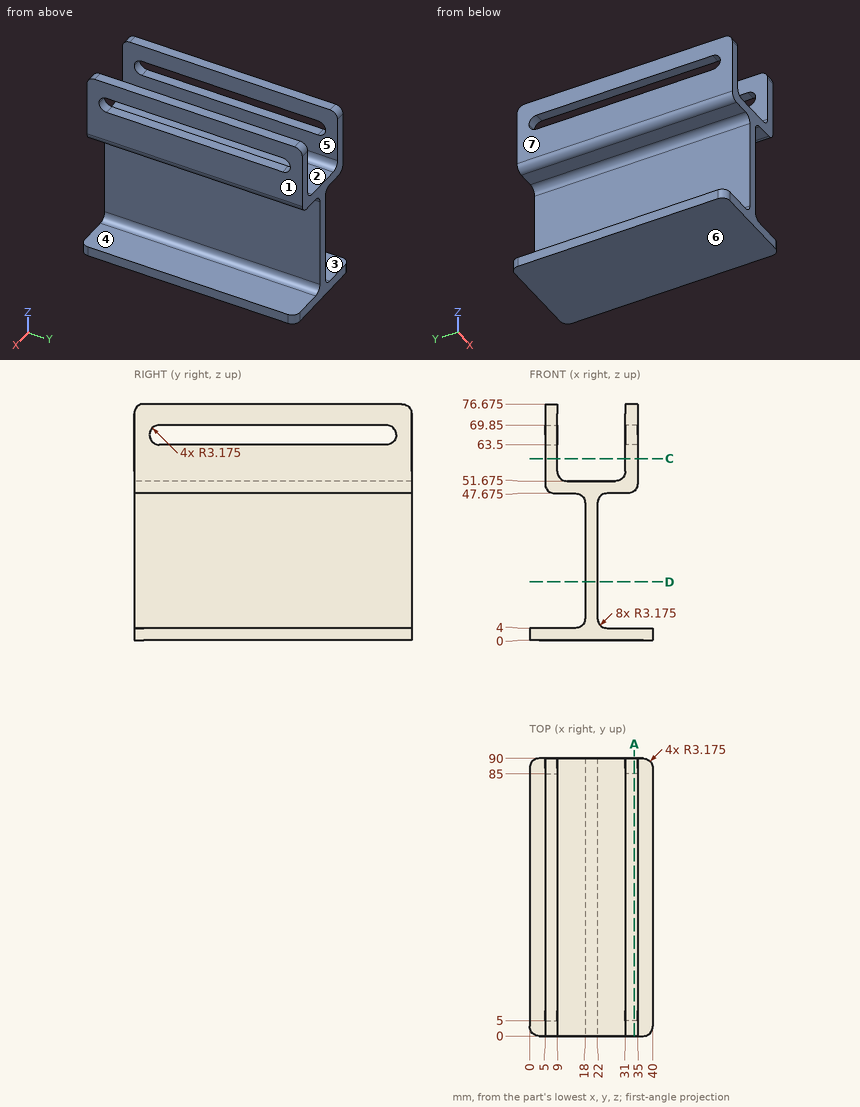
Here's the drawing with two shaded views (mm, measured from the low corner). I have some questions. A direction names the side the tool comes from. Give positions to 0.01 mm unless a question says otherwise; leave off trailing zeros. Loops run counter-clockwise (first coordinate to the right, second up) from the corner with the lowest first, then second, coordinate; pieces in that order, holes last. Notation, with made-up numbers: M 63,84 L 120,84 A12 ccw 120,96 Z; hole C 78.25,-13.5 d3. An arc over 180 degrees is marked long. One line per item, written item: value. Start each with the question number.
1) If we section it at D-D, the plane z = 19: Write out the boundary of the cut face in (x, y).
2) If I drill on line 1 (X direction, y = 19, z = 57); line 2 (Z direction, x = 27, y = 66) (3 decimals); line 3 (Z direction, x = 5.5, y = 29) (3 decimals), over which ranges is the centre line in solid material (lowest first)? Write a range as [from, to].
3) If we section it at A-A, the plane x = 34: Give the number of separate pieces and of enclosed holes in the cut face, and give its area (3 significant figures).
4) I'm going to push flat-ended pins straight in: pin 1 (5 mm diameter, centred on y = 59.5, z = 29, fed in from -X); pin 2 (10 mm diameter, centred on x = 32, y = 55.5, fed in from -Z); pin 3 (4 mm diameter, centred on y = 52, z = 10, fed in from +X); pin 4 (2 mm diameter, centred on x = 12, y = 24.5, fed in from +Z). Where does each tip first touch, or does it pass through?
5) Thinking about a two-plate mould opening in X: for the marked faces 5, 6 and 7, which applies, +X half, -X half, draft (parallel to the pull), parting line (faces both ways), or undercut?
6) If we section it at C-C, the plane z = 59: Write out the boundary of the cut face in (x, y), and give its area (3 significant figures).
7) On a 3-axis mill with a long thin cutter (end or side, diameter ignored), from which of +Z, -Z, +X, -X, +Y, -Y can I reach the whole of each face in a straight line? I mean the marked faces 1, 2, 3 and 4. Say none if no direction works.
Completed:
1. outline: M 18,0 L 22,0 L 22,90 L 18,90 Z
2. line 1: x = [5, 9], [31, 35]
2. line 2: z = [0, 4], [47.675, 51.675]
2. line 3: z = [0, 4], [49.14, 63.5], [69.85, 76.675]
3. separate pieces: 2
3. enclosed holes: 1
3. area: 2,390 mm^2
4. pin 1: stops at x = 18
4. pin 2: stops at z = 0
4. pin 3: stops at x = 22
4. pin 4: stops at z = 51.9
5. face 5: undercut
5. face 6: draft
5. face 7: -X half
6. outline: M 5,0 L 9,0 L 9,90 L 5,90 Z; M 31,0 L 35,0 L 35,90 L 31,90 Z
6. area: 720 mm^2
7. face 1: +Z, +X, +Y, -Y
7. face 2: +Z, +Y, -Y
7. face 3: -X, +Y, -Y
7. face 4: +X, +Y, -Y
